Autodesk Inventor part; units mm, degrees
ref_plane "YZ Plane" through (0, 0, 0) normal (1, 0, 0) x (0, 1, 0)
ref_plane "XZ Plane" through (0, 0, 0) normal (0, 1, 0) x (-1, 0, 0)
ref_plane "XY Plane" through (0, 0, 0) normal (0, 0, 1) x (1, 0, 0)
sketch "Sketch1" plane through (0, 0, 0) normal (0, 0, 1) x (1, 0, 0)
  line L0 (0, 0) -> (19.05, 0)
  line L1 (19.05, 0) -> (19.05, 19.05)
  line L2 (19.05, 19.05) -> (0, 19.05)
  line L3 (0, 19.05) -> (0, 0)
  line L4 (17.4625, 17.4625) -> (1.5875, 17.4625)
  line L5 (1.5875, 17.4625) -> (1.5875, 1.5875)
  line L6 (1.5875, 1.5875) -> (17.4625, 1.5875)
  line L7 (17.4625, 1.5875) -> (17.4625, 17.4625)
  dimension "d0" = 19.05
  dimension "d1" = 19.05
  dimension "d2" = 1.5875
  dimension "d3" = 1.5875
  dimension "d4" = 1.5875
  dimension "d5" = 1.5875
extrude "Extrusion1" add sketch "Sketch1" along normal blind 673.1
sketch "Sketch2" plane through (0, 19.05, 0) normal (0, 1, 0) x (1, 0, 0)
  line L0 (19.05, 0) -> (0, 0)
  line L1 (0, 0) -> (0, -673.1)
  line L2 (19.05, -673.1) -> (0, -673.1)
  line L3 (19.05, -673.1) -> (0, -654.05)
  line L4 (19.05, 0) -> (0, -19.05)
  dimension "d8" = 45
  dimension "d9" = 45
extrude "Extrusion2" cut sketch "Sketch2" against normal through all
equation "\"d3\" = d2"
equation "\"d4\" = d2"
equation "\"d5\" = d3"
properties part number "Bumper Rail Side"
Geometry check sheet. Reference: the model listing, model coordinates, mm. A direction names the side the tool comes from. Coordinates: 2 decimals unless noted, no trailing zeros. Loops run counter-clockwise (first coordinate to the right, second up) from the corner with the lowest first, then second, coordinate; pieces in that order, holes last.
Item 1: Sectioned sample at B-B, the plane z = 630.5. Record the boundary of the cut face in (x, y), then the cut area to 3 significant figures.
Item 2: Thickness scan on line 1 (Y direction, x = 13, z = 388); line 2 (Z direction, x = 9.75, y = 1.5). Record the ranges inside material, lowest first.
Item 3: Sectioned sample at A-A, the plane x = 12. Record the boundary of the cut face in (y, z).
Item 4: Access from +Z, -Z, +X, -X, +Y, -Y to the whole of each face (thin tool, end or side, straight path). Record for faces 5 (the face through (19.05, 9, 332)), 6 (the face through (10, 17.462, 332)).
Item 5: Go/stop test with a flat-tipped pin: pin 1 Ø6 at (x, y) = (7.5, 16.5) entering from +Z. Record where the tip stops, or that it passes through.
Item 6: Sectioned sample at C-C, the plane y = 6.5. Record the boundary of the cut face in (x, z), then the cut area to 3 significant figures.
Item 7: Release check for a two-part mould opening along Y. For faces 1 (the face through (9.66, 18.13, 9.39)), 2 (the face through (9, 0, 332)), 3 (the face through (10, 19.05, 332)), 4 (the face through (1.588, 10, 332)) record: released by +Y, released by -Y, zero draft, split by the parting line, or undercut.
Check result:
1. outline: (0, 0) - (19.05, 0) - (19.05, 19.05) - (0, 19.05) - close; hole (1.59, 1.59) - (17.46, 1.59) - (17.46, 17.46) - (1.59, 17.46) - close
1. area: 111 mm2
2. line 1: y = 0 to 1.59, 17.46 to 19.05
2. line 2: z = 9.3 to 663.8
3. outline: (0, 7.05) - (1.59, 7.05) - (1.59, 666.05) - (0, 666.05) - close; (17.46, 7.05) - (19.05, 7.05) - (19.05, 666.05) - (17.46, 666.05) - close
4. face 5: +Z, -Z, +X, +Y, -Y
4. face 6: +Z, -Z
5. pin 1: stops at z = 664.39
6. outline: (0, 19.05) - (1.59, 17.46) - (1.59, 655.64) - (0, 654.05) - close; (17.46, 1.59) - (19.05, 0) - (19.05, 673.1) - (17.46, 671.51) - close
6. area: 2,080 mm2
7. face 1: zero draft
7. face 2: released by -Y
7. face 3: released by +Y
7. face 4: undercut
